Study the drawing (mm; zero at the part's minimum x, y, z) and answer. A direction names the side the tool comes from. Give positions to 0.01 mm unless a question says otherwise; leave off trailing zeros. Write each loop counter-clockwise with the first axis right and the second up, starting at its lowest first coordinate (ties: lowest second). Pieces come first, ordered by that corner, then holes. Notation, with made-up numbers: M 63,30 L 89,30 A21 cw 89,45 Z; hole C 77,74.5 d7. An arc over 180 degrees is marked long. Use a Markdown table: item, result. Add a question column.
Item 1: A cutting plane is placed at D-D on x = 4.5. Determine the outline of the cut face in (y, z), then the cut area to 3 significant figures.
Item 2: For the marked faces 1 and 2, determine the directions among +Z, -Z, +X, -X, +Y, -Y from which every point of the face is accessible in a straight line to the end or side of a thin tool.
Item 3: Given P1, Ø2, axis at x = 4.5, y = 1.5, coming from the -Z side, flat-ended and moving along its own axis, determine where the tip first touches the part or whether it passes through.
Item 4: A cutting plane is placed at A-A on x = 2. Determine the outline of the cut face in (y, z) (1 decimal).
Item 5: A cutting plane is placed at C-C on z = 1. Determine the outline of the cut face in (x, y).
Item 6: Consider probe 1 along Y at (x, z) = (5, 3); probe 2 along X at (y, z) = (3.4, 3); probe 3 along X at (y, z) = (2.85, 3.25) (1 decimal). Determine where each line is inside the solid, lowest interval first. Write a range as [from, to].
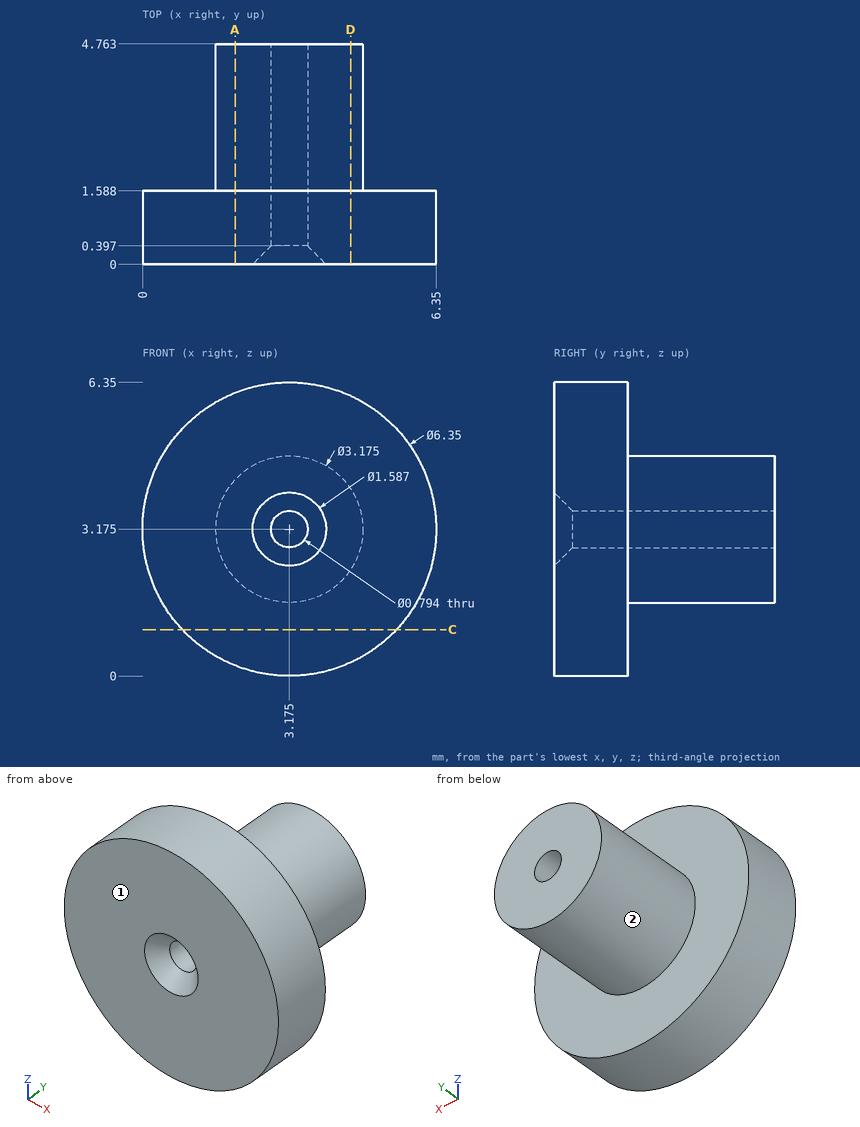
Filled in:
| question | item | result |
|---|---|---|
| 1 | outline | M 0,0.29 L 1.59,0.29 L 1.59,2.3 L 4.76,2.3 L 4.76,4.05 L 1.59,4.05 L 1.59,6.06 L 0,6.06 Z |
| 1 | area | 14.7 mm² |
| 2 | face 1 | +Z, -Z, +X, -X, -Y |
| 2 | face 2 | +Y |
| 3 | P1 | z = 0.02 |
| 4 | outline | M 0,0.2 L 1.6,0.2 L 1.6,2.1 L 4.8,2.1 L 4.8,4.2 L 1.6,4.2 L 1.6,6.1 L 0,6.1 Z |
| 5 | outline | M 0.86,0 L 5.49,0 L 5.49,1.59 L 0.86,1.59 Z |
| 6 | probe 1 | [0, 1.59] |
| 6 | probe 2 | [1.6, 2.82], [3.53, 4.75] |
| 6 | probe 3 | [1.6, 2.8], [3.6, 4.8] |
